Geometry: final body of the model. Coordinates: model frame, mm. A direction names the side the tool comes from. Coordinates: 2 decimals unless noted, no trailing zeros. Order: outer loops, then holes, each group sorted by start corner. A loop starts at its lowest first (then second) coordinate and runs counter-clockwise, first axis right, second up. Notation, with made-up numbers: (-4.5, -8) -> (1.5, -8) arc R25 ccw to (1.5, 31) -> close; hole circle Ø4 at (77.25, 0). An arc over 180 degrees is marked (long way). Answer in a Markdown table with one row per item. Add a question column.
1) Section query C-C on x = -158. Return the cut outline in (y, z), then the cut area to 3 significant figures.
2) Section query B-B on x = -90. Return the cut outline in (y, z), then the cut area to 3 significant figures.
3) Pull-direction query (X, two-part tool) for faces 3 (the face through (-166.92, 183.58, 1.48)), 4 (the face through (-215, 3, 3)), 5 (the face through (-245.98, 120.68, 1.48)), 6 (the face through (-64.174, -160.043, 1.479)); classes: +X half, -X half, draft (parallel to the pull), parting line (faces both ways), or undercut.
4) Section query D-D on y = -107. Return the cut outline in (x, z).
5) Ray query, line 1 (Y direction, x = -155, z = 1.05); line 2 (Y direction, x = -213, z = 2.15); line 3 (X direction, y = 113, z = 1.95). Return the intervals inside material, ascending. Write a range as from..to.
6) Contact query for flat-ended pins moving along their axis: P1, Ø1.5, axis at x = -106.5, z = 2.5, coming from the -Y side; P2, Ø0.9, axis at x = -470, z = 1, coming from the +Y side; P3, Ø1.5, axis at x = -470.5, z = 1, coming from the -Y side. Output: stop coordinate, or through.
7) Section query A-A on y = 126.5. Return the cut outline in (x, z), then the cut area to 3 significant figures.
8) Set-up query: faces 1 (the face through (-132.06, -73.036, 1.479)), 2 (the face through (-215, 3, 0)). Return all of +Z, -Z, +X, -X, +Y, -Y with unobstructed straight access to the full face (end or side cutting, diameter ignored); none if empty.
Autodesk Inventor part; units mm, degrees
ref_plane "Work Plane1" through (0, 0, 0) normal (0, 0, 1) x (1, 0, 0)
ref_plane "YZ Plane" through (0, 0, 0) normal (1, 0, 0) x (0, 1, 0)
ref_plane "XZ Plane" through (0, 0, 0) normal (0, 1, 0) x (-1, 0, 0)
ref_plane "Work Plane1" through (0, 0, 0) normal (0, 0, 1) x (1, 0, 0)
sketch "Sketch1" plane through (0, 0, 0) normal (0, 0, 1) x (1, 0, 0)
  line L0 (-79.5271, 221.8978) -> (-38.5876, 0.7641) construction
  line L1 (-214.8536, 60) -> (-51.8859, 87.6696)
  line L2 (-53.5598, 97.5285) -> (-216.5275, 69.8589)
  line L3 (-216.5275, 69.8589) -> (-214.8536, 60)
  line L4 (-265.8796, 142.5897) -> (-244.8522, 91.8249)
  line L5 (-235.6134, 95.6518) -> (-256.6408, 146.4165)
  line L6 (-235.6134, 95.6518) -> (-244.8522, 91.8249)
  line L7 (-413.7003, -81.3604) -> (-404.4616, -85.1872) construction
  line L8 (-392.6729, -30.5956) -> (-413.7003, -81.3604)
  line L9 (-404.4616, -85.1872) -> (-383.4341, -34.4224)
  line L10 (-244.8727, -91.8744) -> (-265.9001, -142.6392)
  line L11 (-265.9001, -142.6392) -> (-256.6613, -146.466) construction
  line L12 (-256.6613, -146.466) -> (-235.6339, -95.7013)
  line L13 (-486.3009, 5) -> (-486.3009, -5) construction
  line L14 (-486.3009, -5) -> (-431.3536, -5)
  line L15 (-431.3536, 5) -> (-486.3009, 5)
  line L16 (-431.3536, 5) -> (-431.3536, -5)
  line L17 (-411.8071, 76.7896) -> (-402.5683, 80.6164) construction
  line L18 (-411.8071, 76.7896) -> (-390.7796, 26.0248)
  line L19 (-381.5408, 29.8516) -> (-402.5683, 80.6164)
  line L20 (-390.7796, 26.0248) -> (-381.5408, 29.8516)
  line L21 (-256.6408, 146.4165) -> (-265.8796, 142.5897) construction
  line L22 (-167.233, 78.2284) -> (-53.5598, 97.5285)
  line L23 (-51.8859, 87.6696) -> (-165.5591, 68.3695)
  line L24 (-53.5598, 97.5285) -> (-51.8859, 87.6696) construction
  line L25 (-51.7174, -86.6773) -> (-214.6851, -59.0077)
  line L26 (-51.7174, -86.6773) -> (-53.3913, -96.5362) construction
  line L27 (-216.359, -68.8666) -> (-53.3913, -96.5362)
  line L28 (-214.6851, -59.0077) -> (-216.359, -68.8666)
  line L29 (-392.6729, -30.5956) -> (-383.4341, -34.4224)
  line L30 (-244.8727, -91.8744) -> (-235.6339, -95.7013)
  line L31 (-481.3536, 5) -> (-431.3536, 5)
  line L32 (-486.3009, -51.2882) -> (-413.7003, -81.3604)
  line L33 (-486.3009, -51.2882) -> (-486.3009, -5)
  line L34 (-486.3009, 5) -> (-486.3009, 51.2882)
  line L35 (-256.6408, 146.4165) -> (-74.6586, 221.796)
  line L36 (-37.0008, 0) -> (-51.8859, 87.6696)
  line L37 (-53.5598, 97.5285) -> (-74.6586, 221.796)
  line L38 (-74.6586, -221.796) -> (-53.3913, -96.5362)
  line L39 (-51.7174, -86.6773) -> (-37.0008, 0)
  line L40 (-404.4616, -85.1872) -> (-265.8796, -142.5897)
  line L41 (-256.6408, -146.4165) -> (-74.6586, -221.796)
  line L42 (-411.8071, 76.7896) -> (-413.7003, 81.3604)
  line L43 (-402.5683, 80.6164) -> (-404.4616, 85.1872)
  line L44 (-486.3009, 51.2882) -> (-413.7003, 81.3604)
  line L45 (-404.4616, 85.1872) -> (-265.8796, 142.5897)
  point P0 (0, 0)
extrude "Extrusion1" add sketch "Sketch1" along normal blind 3
properties part number "refbot" material "Wood (Cherry)"
Result:
| question | item | result |
|---|---|---|
| 1 | outline | (-187.27, 0) -> (-78.78, 0) -> (-78.78, 3) -> (-187.27, 3) -> close; (-68.63, 0) -> (69.65, 0) -> (69.65, 3) -> (-68.63, 3) -> close; (79.8, 0) -> (187.27, 0) -> (187.27, 3) -> (79.8, 3) -> close |
| 1 | area | 1,060 mm2 |
| 2 | outline | (-215.44, 0) -> (-90.32, 0) -> (-90.32, 3) -> (-215.44, 3) -> close; (-80.18, 0) -> (81.2, 0) -> (81.2, 3) -> (-80.18, 3) -> close; (91.34, 0) -> (215.44, 0) -> (215.44, 3) -> (91.34, 3) -> close |
| 2 | area | 1,230 mm2 |
| 3 | face 3 | -X half |
| 3 | face 4 | draft |
| 3 | face 5 | undercut |
| 3 | face 6 | +X half |
| 4 | outline | (-351.8, 0) -> (-251.14, 0) -> (-251.14, 3) -> (-351.8, 3) -> close; (-240.31, 0) -> (-55.17, 0) -> (-55.17, 3) -> (-240.31, 3) -> close |
| 5 | line 1 | -188.52..-79.28, -69.14..70.16, 80.31..188.52 |
| 5 | line 2 | -164.49..-69.44, -59.29..60.31, 70.46..164.49 |
| 5 | line 3 | -337.32..-253.62, -242.8..-56.19 |
| 6 | P1 | y = -208.92 |
| 6 | P2 | y = 58.23 |
| 6 | P3 | y = -58.14 |
| 7 | outline | (-304.72, 0) -> (-259.22, 0) -> (-259.22, 3) -> (-304.72, 3) -> close; (-248.39, 0) -> (-58.48, 0) -> (-58.48, 3) -> (-248.39, 3) -> close |
| 7 | area | 706 mm2 |
| 8 | face 1 | +Z, -Z |
| 8 | face 2 | -Z, +X, -X, +Y, -Y |
